For this review, use the dimensioned drawing (mm, ordinates from the lowest corner) and the shaded views. A direction names the side the tool comes from. Coordinates: 2 decimals unless noted, no trailing zeros. Write each loop counter-clockwise with the first axis right and the second up, starting at its lowest first coordinate (ties: lowest second). Pieces come first, ordered by that corner, then holes.
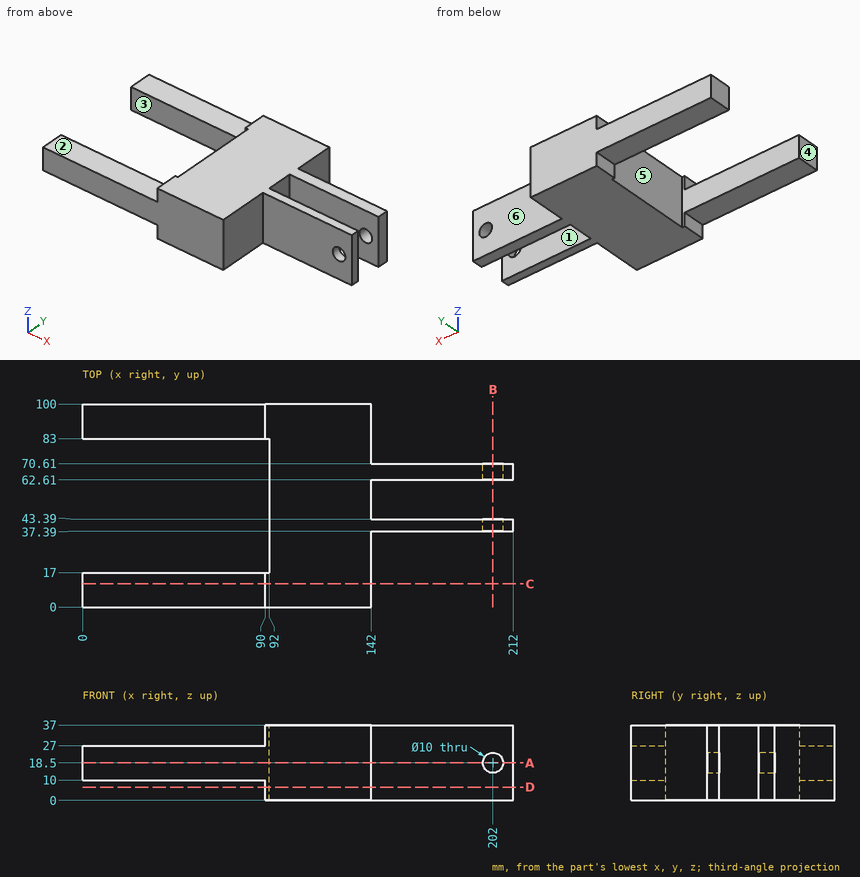
Item 1: Take a section at D-D, the plane z = 6.5. Write out the cut boundary in (x, y).
Solved:
outline: (90, 0) - (142, 0) - (142, 37.39) - (212, 37.39) - (212, 43.39) - (142, 43.39) - (142, 62.61) - (212, 62.61) - (212, 70.61) - (142, 70.61) - (142, 100) - (90, 100) - (90, 83) - (92, 83) - (92, 17) - (90, 17) - close
Item 2: For pin 1 (8 mm diameter, centred on y = 88, z = 4.5, fed in from -X); pin 2 (13.5 mm diameter, centred on x = 57, y = 5, fed in from +Z); pin 3 (5 mm diameter, centred on y = 29, z = 28, fed in from +X), all flat-tipped, find the tip position at first contact; note any pin that passes through.
Solved:
pin 1: stops at x = 90
pin 2: stops at z = 27
pin 3: stops at x = 142
Item 3: Mouldability with a two-part tool opening along Y and no side actions: class the marked faces 4, 5 and 6 as pulls with the +Y half, pulls with the -Y half, needs draft (parallel to the pull), parting line crosses it, or undercut.
Solved:
face 4: needs draft
face 5: undercut
face 6: pulls with the +Y half
Item 4: To check wall thickness, follow line 1 along X through (y, z) = (39.85, 18.5); line 2 along Y through (x, z) = (155, 26.5); line 3 along Z through (x, y) = (202, 67). State the ranges of each line that lie inside material, in increasing order.
Solved:
line 1: x = 92 to 197, 207 to 212
line 2: y = 37.39 to 43.39, 62.61 to 70.61
line 3: z = 0 to 13.5, 23.5 to 37
Item 5: Machinability: for the marked faces 1, 2 and 3, which of the approach directions +Z, -Z, +X, -X, +Y, -Y give a long, thin tool a straight path to every point of the face, cutting with its end or side? Answer none if there is none.
Solved:
face 1: +Z, -Z, +X
face 2: +Z, -X, +Y, -Y
face 3: +Z, -Z, -X
Item 6: Take a section at C-C, the plane y = 11.5. Write out the cut boundary in (x, z), plus the area to 3 significant figures.
Solved:
outline: (0, 10) - (90, 10) - (90, 0) - (142, 0) - (142, 37) - (90, 37) - (90, 27) - (0, 27) - close
area: 3,450 mm2
Item 7: Take a section at B-B, the plane x = 202. Write out the cut boundary in (y, z), plus the area to 3 significant figures.
Solved:
outline: (37.39, 0) - (43.39, 0) - (43.39, 13.5) - (37.39, 13.5) - close; (37.39, 23.5) - (43.39, 23.5) - (43.39, 37) - (37.39, 37) - close; (62.61, 0) - (70.61, 0) - (70.61, 13.5) - (62.61, 13.5) - close; (62.61, 23.5) - (70.61, 23.5) - (70.61, 37) - (62.61, 37) - close
area: 378 mm2
Item 8: Take a section at A-A, the plane z = 18.5. Write out the cut boundary in (x, y), plus the area to 3 significant figures.
Solved:
outline: (0, 0) - (142, 0) - (142, 37.39) - (197, 37.39) - (197, 43.39) - (142, 43.39) - (142, 62.61) - (197, 62.61) - (197, 70.61) - (142, 70.61) - (142, 100) - (0, 100) - (0, 83) - (92, 83) - (92, 17) - (0, 17) - close; (207, 37.39) - (212, 37.39) - (212, 43.39) - (207, 43.39) - close; (207, 62.61) - (212, 62.61) - (212, 70.61) - (207, 70.61) - close
area: 8,970 mm2
